```python
from build123d import *

# Parameters (mm, degrees)
BOSS_EXTRUDE1_DEPTH = 25.4
SKETCH5_W           = 1.5875
SKETCH5_H           = 15.37716
BOSS_EXTRUDE3_DEPTH = 15.24


with BuildPart() as part:
    # Sketch1 → Boss-Extrude1 (new body)
    with BuildSketch(Plane(origin=(0, 0, 0), x_dir=(1, 0, 0), z_dir=(0, 1, 0))):
        Polygon((38.1, 63.5), (28.9941, 63.5), (-28.9941, 63.5), (-38.1, 63.5), (-38.1, -63.5), (38.1, -63.5), align=None)
    extrude(amount=BOSS_EXTRUDE1_DEPTH)

    # Sketch5 → Boss-Extrude3 (add)
    with BuildSketch(Plane(origin=(0, 0, -63.5), x_dir=(-1, 0, 0), z_dir=(0, 0, -1))):
        with Locations((-28.20035, 7.68858)):
            Rectangle(SKETCH5_W, SKETCH5_H)
        with Locations((26.42680374, 7.68858)):
            Rectangle(SKETCH5_W, SKETCH5_H)
    extrude(amount=BOSS_EXTRUDE3_DEPTH)


solid = part.part
```
Geometry: final body of the model. Coordinates: model frame, mm. A direction names the side the tool comes from. Coordinates: 2 decimals unless noted, no trailing zeros. Loops run counter-clockwise (first coordinate to the right, second up) from the corner with the lowest first, then second, coordinate; pieces in that order, holes last. Notation, with made-up numbers: M -25,3 L 22,3 A28 ccw 22,21 Z; hole C 41.25,-10.75 d11. An arc over 180 degrees is marked long. Put each result on its own line as item: value.
(1) Access query for faces 1 (the face through (28.994, 8, -71)), 2 (the face through (-1, 25.4, -1)), 3 (the face through (-25.633, 8, -71)). Directions: +Z, -Z, +X, -X, +Y, -Y. A direction counts if a zero-diameter tool reaches every point of the face in a straight line with its end or side. Return the directions, or none.
Answer sheet:
face 1: -Z, +X, +Y, -Y
face 2: +Z, -Z, +X, -X, +Y
face 3: -Z, +Y, -Y
(2) Material intervals for probe 1 along X at (y, z) = (14.75, -66); probe 2 along Z at (x, y) = (-31, 3.25), sorted ascending.
Answer sheet:
probe 1: x = -27.22 to -25.63, 27.41 to 28.99
probe 2: z = -63.5 to 63.5
(3) Cut plane A-A on z = -69.5. Return the cut outline in (x, y), then the cut area to 3 significant figures.
Answer sheet:
outline: M -27.22,0 L -25.63,0 L -25.63,15.38 L -27.22,15.38 Z; M 27.41,0 L 28.99,0 L 28.99,15.38 L 27.41,15.38 Z
area: 48.8 mm^2
(4) First-contact query: pin 1 (7.5 mm diameter, centred on y = 5, z = -72.5, fed in from +X); pin 2 (0.5 mm diameter, centred on x = 28, z = -70.5, fed in from +Y); pin 3 (2 mm diameter, centred on x = 26, y = 10.5, fed in from -Z). Flat tips, straight axial feed; report the tip coordinate or a pass-through.
Answer sheet:
pin 1: stops at x = 28.99
pin 2: stops at y = 15.38
pin 3: stops at z = -63.5
(5) Draft query along X for faces 4 (the face through (-27.221, 8, -71)), 5 (the face through (-1, 13, 63.5)), 6 (the face through (1, 13, -63.5)), 7 (the face through (38.1, 13, 1)). Return one class per face: pulls with the +X half, pulls with the -X half, needs draft (parallel to the pull), parting line crosses it, or undercut.
Answer sheet:
face 4: pulls with the -X half
face 5: needs draft
face 6: undercut
face 7: pulls with the +X half
(6) Cut plane D-D on y = 23.5. Return the cut outline in (x, z), then the cut area to 3 significant figures.
Answer sheet:
outline: M -38.1,-63.5 L 38.1,-63.5 L 38.1,63.5 L -38.1,63.5 Z
area: 9,680 mm^2
(7) Cut plane B-B on y = 8.25. Return the cut outline in (x, z).
Answer sheet:
outline: M -38.1,-63.5 L -27.22,-63.5 L -27.22,-78.74 L -25.63,-78.74 L -25.63,-63.5 L 27.41,-63.5 L 27.41,-78.74 L 28.99,-78.74 L 28.99,-63.5 L 38.1,-63.5 L 38.1,63.5 L -38.1,63.5 Z
(8) Cut plane C-C on x = -17. Return the cut outline in (y, z), then the cut area to 3 significant figures.
Answer sheet:
outline: M 0,-63.5 L 25.4,-63.5 L 25.4,63.5 L 0,63.5 Z
area: 3,230 mm^2
